Can you work these out from the model? Positions are in its coordinate system, mm. Coordinates: 2 decimals unless noted, no trailing zeros. Order: outer loops, then holes, each group sorted by start corner. A loop starts at its lowest first (then second) coordinate and runs counter-clockwise, first axis right, second up. Notation, with made-up numbers: (63, 66.25) -> (105, 66.25) arc R31 cw to (105, 91.25) -> close; hole circle Ø9 at (45, 51). An arc over 180 degrees is marked (long way). Use a Markdown table: item, result. Add a question column.
1. If I drill on line 1 along X through (y, z) = (28, 2.85); line 2 along Y through (x, z) = (189.5, 2.1); line 3 along Y through (x, z) = (147, 1.85), over which ranges is the centre line in solid material (lowest first)? Write a range as from..to.
2. Suppose I cut it at C-C, the plane x = 422.5. List the corners of the cut face in (y, z) for me.
3. Suppose I cut it at A-A, the plane x = 313.5. List the corners of the cut face in (y, z) for me.
4. Suppose I cut it at D-D, the plane z = 1.85. State how many separate pieces and enclosed holes the cut face has, then the cut area to 3 significant figures.
5. Suppose I cut it at B-B, the plane y = 111.5. List the corners of the cut face in (x, z) for me, then the cut area to 3 significant figures.
Autodesk Inventor part; units mm, degrees
ref_plane "YZ Plane" through (0, 0, 0) normal (1, 0, 0) x (0, 1, 0)
ref_plane "XZ Plane" through (0, 0, 0) normal (0, 1, 0) x (-1, 0, 0)
ref_plane "XY Plane" through (0, 0, 0) normal (0, 0, 1) x (1, 0, 0)
sketch "Boceto1" plane through (0, 0, 0) normal (0, 0, 1) x (1, 0, 0)
  line L0 (0, 0) -> (0, 210)
  line L1 (0, 210) -> (450, 210)
  line L2 (450, 210) -> (450, 0)
  line L3 (450, 0) -> (0, 0)
  line L4 (5, 5) -> (5, 35.71)
  line L5 (5, 5) -> (50, 5)
  line L6 (50, 5) -> (50, 8)
  line L7 (5, 35.71) -> (8, 35.71)
  line L8 (50, 8) -> (8, 8)
  line L9 (8, 8) -> (8, 35.71)
  line L10 (5, 63.43) -> (5, 91.14)
  line L11 (5, 118.86) -> (5, 146.57)
  line L12 (5, 174.29) -> (5, 205)
  line L13 (5, 205) -> (50, 205)
  line L14 (5, 63.43) -> (8, 63.43)
  line L15 (8, 63.43) -> (8, 91.14)
  line L16 (8, 91.14) -> (5, 91.14)
  line L17 (5, 118.86) -> (8, 118.86)
  line L18 (8, 118.86) -> (8, 146.57)
  line L19 (8, 146.57) -> (5, 146.57)
  line L20 (50, 205) -> (50, 202)
  line L21 (5, 174.29) -> (8, 174.29)
  line L22 (8, 174.29) -> (8, 202)
  line L23 (8, 202) -> (50, 202)
  line L24 (100, 205) -> (150, 205)
  line L25 (200, 205) -> (250, 205)
  line L26 (300, 205) -> (350, 205)
  line L27 (400, 205) -> (445, 205)
  line L28 (445, 205) -> (445, 174.29)
  line L29 (100, 205) -> (100, 202)
  line L30 (100, 202) -> (150, 202)
  line L31 (150, 202) -> (150, 205)
  line L32 (200, 205) -> (200, 202)
  line L33 (200, 202) -> (250, 202)
  line L34 (250, 202) -> (250, 205)
  line L35 (300, 205) -> (300, 202)
  line L36 (300, 202) -> (350, 202)
  line L37 (350, 202) -> (350, 205)
  line L38 (400, 205) -> (400, 202)
  line L39 (445, 174.29) -> (442, 174.29)
  line L40 (442, 174.29) -> (442, 202)
  line L41 (442, 202) -> (400, 202)
  line L42 (445, 146.57) -> (445, 118.86)
  line L43 (445, 91.14) -> (445, 63.43)
  line L44 (445, 35.71) -> (445, 5)
  line L45 (445, 5) -> (400, 5)
  line L46 (445, 35.71) -> (442, 35.71)
  line L47 (400, 5) -> (400, 8)
  line L48 (400, 8) -> (442, 8)
  line L49 (442, 8) -> (442, 35.71)
  line L50 (445, 63.43) -> (442, 63.43)
  line L51 (442, 63.43) -> (442, 91.14)
  line L52 (442, 91.14) -> (445, 91.14)
  line L53 (445, 118.86) -> (442, 118.86)
  line L54 (442, 118.86) -> (442, 146.57)
  line L55 (442, 146.57) -> (445, 146.57)
  line L56 (100, 5) -> (150, 5)
  line L57 (200, 5) -> (250, 5)
  line L58 (300, 5) -> (350, 5)
  line L59 (100, 5) -> (100, 8)
  line L60 (100, 8) -> (150, 8)
  line L61 (150, 8) -> (150, 5)
  line L62 (200, 5) -> (200, 8)
  line L63 (200, 8) -> (250, 8)
  line L64 (250, 8) -> (250, 5)
  line L65 (300, 5) -> (300, 8)
  line L66 (300, 8) -> (350, 8)
  line L67 (350, 8) -> (350, 5)
  line L68 (225, 174.29) -> (326.5, 174.29)
  line L69 (225, 174.29) -> (123.5, 174.29)
  line L70 (326.5, 174.29) -> (326.5, 87.29)
  line L71 (326.5, 87.29) -> (123.5, 87.29)
  line L72 (123.5, 87.29) -> (123.5, 174.29)
  line L73 (225, 52) -> (326.5, 52)
  line L74 (225, 52) -> (123.5, 52)
  line L75 (123.5, 52) -> (123.5, 66.5)
  line L76 (123.5, 66.5) -> (326.5, 66.5)
  line L77 (326.5, 66.5) -> (326.5, 52)
  line L78 (48, 146.57) -> (63, 146.57)
  line L79 (63, 146.57) -> (63, 133.57)
  line L80 (63, 133.57) -> (48, 133.57)
  line L81 (48, 133.57) -> (48, 146.57)
  dimension "d0" = 210
  dimension "d1" = 450
  dimension "d2" = 30.71
  dimension "d3" = 45
  dimension "d4" = 3
  dimension "d5" = 3
  dimension "d7" = 27.71
  dimension "d8" = 27.72
  dimension "d9" = 27.71
  dimension "d10" = 27.72
  dimension "d12" = 30.71
  dimension "d13" = 45
  dimension "d14" = 27.72
  dimension "d15" = 3
  dimension "d17" = 3
  dimension "d19" = 3
  dimension "d20" = 3
  dimension "d21" = 50
  dimension "d22" = 50
  dimension "d23" = 50
  dimension "d24" = 50
  dimension "d25" = 50
  dimension "d26" = 50
  dimension "d27" = 50
  dimension "d28" = 45
  dimension "d29" = 30.71
  dimension "d30" = 3
  dimension "d31" = 3
  dimension "d33" = 3
  dimension "d35" = 50
  dimension "d36" = 3
  dimension "d37" = 3
  dimension "d38" = 27.72
  dimension "d39" = 27.71
  dimension "d40" = 27.72
  dimension "d41" = 27.71
  dimension "d42" = 27.72
  dimension "d43" = 30.71
  dimension "d44" = 3
  dimension "d45" = 3
  dimension "d46" = 3
  dimension "d47" = 3
  dimension "d48" = 50
  dimension "d49" = 50
  dimension "d50" = 50
  dimension "d51" = 50
  dimension "d52" = 50
  dimension "d53" = 50
  dimension "d54" = 50
  dimension "d55" = 3
  dimension "d56" = 3
  dimension "d58" = 3
  dimension "d59" = 5
  dimension "d60" = 5
  dimension "d61" = 5
  dimension "d62" = 5
  dimension "d63" = 5
  dimension "d64" = 5
  dimension "d65" = 5
  dimension "d66" = 5
  dimension "d67" = 5
  dimension "d68" = 5
  dimension "d69" = 5
  dimension "d70" = 5
extrude "Extrusión1" add sketch "Boceto1" along normal blind 3
properties part number "Frontal Arduino" material "Madera (nogal)"
Worked out:
| question | item | result |
|---|---|---|
| 1 | line 1 | x = 0..5, 8..442, 445..450 |
| 1 | line 2 | y = 0..52, 66.5..87.29, 174.29..210 |
| 1 | line 3 | y = 0..5, 8..52, 66.5..87.29, 174.29..202, 205..210 |
| 2 | outline | (0, 0) -> (5, 0) -> (5, 3) -> (0, 3) -> close; (8, 0) -> (202, 0) -> (202, 3) -> (8, 3) -> close; (205, 0) -> (210, 0) -> (210, 3) -> (205, 3) -> close |
| 3 | outline | (0, 0) -> (5, 0) -> (5, 3) -> (0, 3) -> close; (8, 0) -> (52, 0) -> (52, 3) -> (8, 3) -> close; (66.5, 0) -> (87.29, 0) -> (87.29, 3) -> (66.5, 3) -> close; (174.29, 0) -> (202, 0) -> (202, 3) -> (174.29, 3) -> close; (205, 0) -> (210, 0) -> (210, 3) -> (205, 3) -> close |
| 4 | separate pieces | 1 |
| 4 | enclosed holes | 17 |
| 4 | area | 71,600 mm² |
| 5 | outline | (0, 0) -> (123.5, 0) -> (123.5, 3) -> (0, 3) -> close; (326.5, 0) -> (450, 0) -> (450, 3) -> (326.5, 3) -> close |
| 5 | area | 741 mm² |
